Source: three-view drawing plus pictorial views. Frame: mm from the lowest corner of the part. A direction names the side the tool comes from. Give positions to 0.01 mm unless a question says otherwise; leave off trailing zeros. Loops run counter-clockwise (first coordinate to the right, second up) from the corner with the lowest first, then second, coordinate; pieces in that order, holes last. Notation, with made-up numbers: (-32, 40.5) - (23, 40.5) arc R26 ccw to (23, 76.5) - close; hole circle Ø3 at (28, -4). An arc over 180 degrees is marked (long way). Put each result on its own line as item: value.
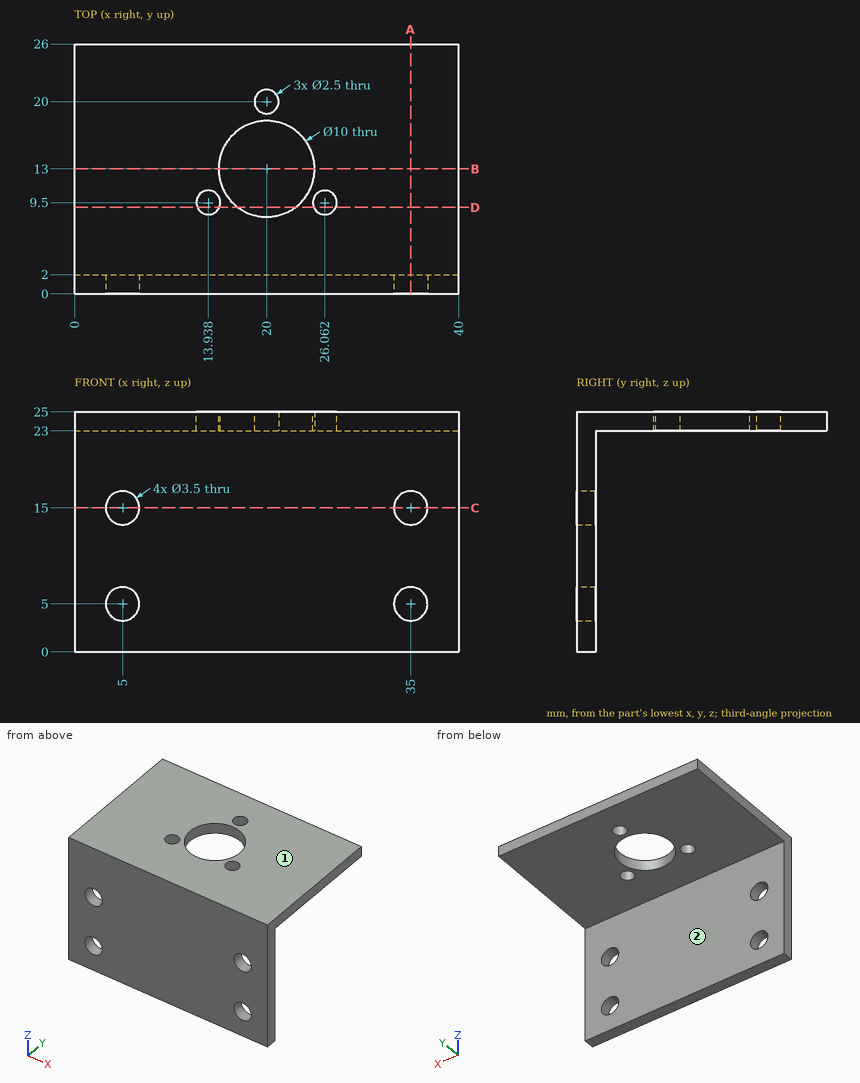
1) Section query D-D, the plane y = 9. Output: boundary loops of the cut face in (x, z).
Check result:
outline: (0, 23) - (12.79, 23) - (12.79, 25) - (0, 25) - close; (15.08, 23) - (17, 23) - (17, 25) - (15.08, 25) - close; (23, 23) - (24.92, 23) - (24.92, 25) - (23, 25) - close; (27.21, 23) - (40, 23) - (40, 25) - (27.21, 25) - close
2) Section query C-C, the plane z = 15. Output: boundary loops of the cut face in (x, y), plus the area to 3 significant figures.
Check result:
outline: (0, 0) - (3.25, 0) - (3.25, 2) - (0, 2) - close; (6.75, 0) - (33.25, 0) - (33.25, 2) - (6.75, 2) - close; (36.75, 0) - (40, 0) - (40, 2) - (36.75, 2) - close
area: 66.0 mm²
3) Material intervals for line 1 along X through (y, z) = (1.5, 15); line 2 along Y through (x, z) = (30.5, 11.5); line 3 along Z through (x, y) = (31, 8.75), sorted ascending. Write a range as [from, to].
Check result:
line 1: [0, 3.25], [6.75, 33.25], [36.75, 40]
line 2: [0, 2]
line 3: [23, 25]
4) Access query for the marked faces 1 and 2. Directions: +Z, -Z, +X, -X, +Y, -Y. A direction counts if a zero-diameter tool reaches every point of the face in a straight line with its end or side. Return the directions, or none.
Check result:
face 1: +Z, +X, -X, +Y, -Y
face 2: -Z, +X, -X, +Y
5) Pin query (flat end, axial travel): P1, Ø12, axis at x = 24.5, y = 17.5, coming from the -Z side; P2, Ø3, axis at x = 5, z = 15, coming from the -Y side; P3, Ø1.5, axis at x = 10, z = 17.5, coming from the +Y side. Return the tip coordinate at first contact, or that it passes through.
Check result:
P1: z = 23
P2: through
P3: y = 2
6) Section query A-A, the plane x = 35. Output: boundary loops of the cut face in (y, z), plus the area to 3 significant figures.
Check result:
outline: (0, 0) - (2, 0) - (2, 3.25) - (0, 3.25) - close; (0, 6.75) - (2, 6.75) - (2, 13.25) - (0, 13.25) - close; (0, 16.75) - (2, 16.75) - (2, 23) - (26, 23) - (26, 25) - (0, 25) - close
area: 84.0 mm²
7) Section query B-B, the plane y = 13. Output: boundary loops of the cut face in (x, z), plus the area to 3 significant figures.
Check result:
outline: (0, 23) - (15, 23) - (15, 25) - (0, 25) - close; (25, 23) - (40, 23) - (40, 25) - (25, 25) - close
area: 60.0 mm²
